Source: CAD feature listing. Evaluate the final solid. Frame: model axes, mm. Face numbers are marked on the shaded views. A direction names the side the tool comes from. Coordinates: 2 decimals unless noted, no trailing zeros. Loops run counter-clockwise (first coordinate to the right, second up) from the corner with the lowest first, then second, coordinate; pieces in that order, holes last. Notation, with made-up numbers: (-24.5, 9) -> (-6.5, 9) arc R34 ccw to (-6.5, 44) -> close; hole circle Ø10 at (34.25, 14). An arc over 180 degrees is marked (long way). Answer as CSV lines item,"result".
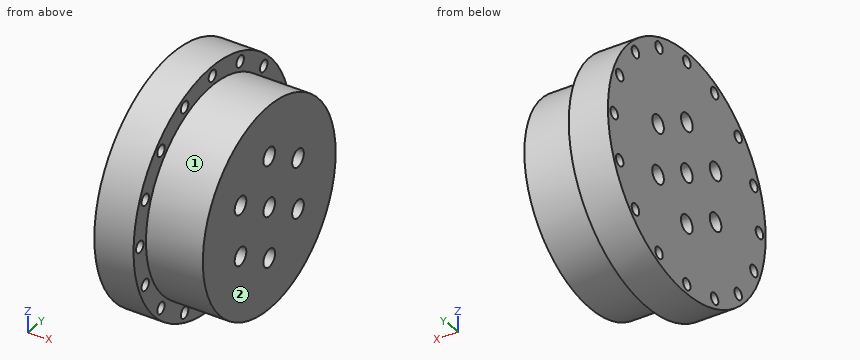
from build123d import *

# Parameters (mm, degrees)
F0_R     = 80
F0_R_2   = 7
F1_DEPTH = 76
F0_R_3   = 95
F0_R_4   = 4.5
F2_DEPTH = 31


with BuildPart() as f1:
    # F0 (on Right) → F1 (new body)
    with BuildSketch(Plane.YZ):
        Circle(F0_R)
        with Locations((-34.641016, -20)):
            Circle(F0_R_2, mode=Mode.SUBTRACT)
        with Locations((0, -40)):
            Circle(F0_R_2, mode=Mode.SUBTRACT)
        with Locations((34.641016, -20)):
            Circle(F0_R_2, mode=Mode.SUBTRACT)
        with Locations((-34.641016, 20)):
            Circle(F0_R_2, mode=Mode.SUBTRACT)
        Circle(F0_R_2, mode=Mode.SUBTRACT)
        with Locations((34.641016, 20)):
            Circle(F0_R_2, mode=Mode.SUBTRACT)
        with Locations((0, 40)):
            Circle(F0_R_2, mode=Mode.SUBTRACT)
    extrude(amount=F1_DEPTH)

    # F0 (on Right) → F2 (join)
    with BuildSketch(Plane.YZ):
        Circle(F0_R_3)
        with Locations((-61.870429, -61.870429)):
            Circle(F0_R_4, mode=Mode.SUBTRACT)
        with Locations((-33.484035, -80.837611)):
            Circle(F0_R_4, mode=Mode.SUBTRACT)
        with Locations((-80.837611, -33.484035)):
            Circle(F0_R_4, mode=Mode.SUBTRACT)
        with Locations((0, -87.498)):
            Circle(F0_R_4, mode=Mode.SUBTRACT)
        with Locations((33.484035, -80.837611)):
            Circle(F0_R_4, mode=Mode.SUBTRACT)
        with Locations((61.870429, -61.870429)):
            Circle(F0_R_4, mode=Mode.SUBTRACT)
        with Locations((80.837611, -33.484035)):
            Circle(F0_R_4, mode=Mode.SUBTRACT)
        with Locations((-87.498, 0)):
            Circle(F0_R_4, mode=Mode.SUBTRACT)
        with Locations((-80.837611, 33.484035)):
            Circle(F0_R_4, mode=Mode.SUBTRACT)
        with Locations((-61.870429, 61.870429)):
            Circle(F0_R_4, mode=Mode.SUBTRACT)
        with Locations((-33.484035, 80.837611)):
            Circle(F0_R_4, mode=Mode.SUBTRACT)
        Circle(F0_R, mode=Mode.SUBTRACT)
        with Locations((87.498, 0)):
            Circle(F0_R_4, mode=Mode.SUBTRACT)
        with Locations((80.837611, 33.484035)):
            Circle(F0_R_4, mode=Mode.SUBTRACT)
        with Locations((0, 87.498)):
            Circle(F0_R_4, mode=Mode.SUBTRACT)
        with Locations((33.484035, 80.837611)):
            Circle(F0_R_4, mode=Mode.SUBTRACT)
        with Locations((61.870429, 61.870429)):
            Circle(F0_R_4, mode=Mode.SUBTRACT)
    extrude(amount=F2_DEPTH)


solid = f1.part
(1) Cut plane B-B (x = 54.5). Return the cut outline in (y, z), then the cut area to 3 significant figures.
Computed values:
outline,"circle Ø160 at (0, 0); hole circle Ø14 at (-34.64, -20); hole circle Ø14 at (-34.64, 20); hole circle Ø14 at (0, -40); hole circle Ø14 at (0, 0); hole circle Ø14 at (0, 40); hole circle Ø14 at (34.64, -20); hole circle Ø14 at (34.64, 20)"
area,"19,000 mm^2"
(2) Cut plane D-D (z = 9.5). Return the cut outline in (x, y), then the cut area to 3 significant figures.
Computed values:
outline,"(0, -94.52) -> (31, -94.52) -> (31, -79.43) -> (76, -79.43) -> (76, 79.43) -> (31, 79.43) -> (31, 94.52) -> (0, 94.52) -> close"
area,"13,000 mm^2"
(3) Pin query (flat end, axial travel): pin 1 Ø10 at (x, y) = (51.5, 66.5) entering from -Z; pin 2 Ø5 at (x, y) = (57, 30) entering from +Z; pin 3 Ø1 at (x, z) = (8.5, -50) entering from +Y. Return the tip coordinate at first contact, or that it passes through.
Computed values:
pin 1,"z = -51.16"
pin 2,"z = 75.12"
pin 3,"y = 81.08"
(4) Material intervals for L1, parallel to Z at x = 47.5, y = -38; L2, parallel to Y at x = 52, z = 17; L3, parallel to Y at x = 28, z = -61.5, sorted ascending. Write a range as [from, to].
Computed values:
L1,"[-70.4, -26.14], [-13.86, 13.86], [26.14, 70.4]"
L2,"[-78.17, -40.97], [-28.32, 28.32], [40.97, 78.17]"
L3,"[-72.41, -66.36], [-57.39, 57.39], [66.36, 72.41]"
(5) Cut plane A-A (y = 0). Return the cut outline in (x, z).
Computed values:
outline,"(0, -95) -> (31, -95) -> (31, -92) -> (0, -92) -> close; (0, -83) -> (31, -83) -> (31, -80) -> (76, -80) -> (76, -47) -> (0, -47) -> close; (0, -33) -> (76, -33) -> (76, -7) -> (0, -7) -> close; (0, 7) -> (76, 7) -> (76, 33) -> (0, 33) -> close; (0, 47) -> (76, 47) -> (76, 80) -> (31, 80) -> (31, 83) -> (0, 83) -> close; (0, 92) -> (31, 92) -> (31, 95) -> (0, 95) -> close"
(6) Cut plane C-C (x = 11). State how many separate pieces and enclosed holes the cut face has, then the cut area to 3 significant figures.
Computed values:
separate pieces,"1"
enclosed holes,"23"
area,"26,300 mm^2"
(7) Access query for the marked faces 1 and 2. Directions: +Z, -Z, +X, -X, +Y, -Y. A direction counts if a zero-diameter tool reaches every point of the face in a straight line with its end or side. Return the directions, or none.
Computed values:
face 1,"+X"
face 2,"+Z, -Z, +X, +Y, -Y"
